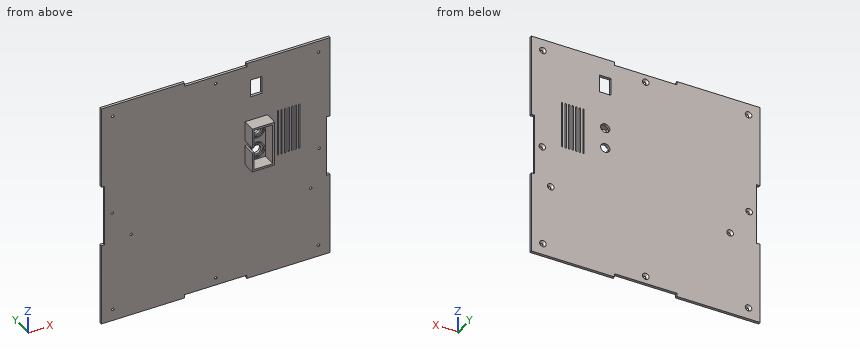
```python
from build123d import *

# Parameters (mm, degrees)
BOSS_EXTRUDE1_DEPTH = 2
SKETCH2_R           = 1
CUT_EXTRUDE1_DEPTH  = 123.699327627
CHAMFER1_SIZE       = 1.5
CUT_EXTRUDE3_DEPTH  = 123.699327627
SKETCH3_W           = 9
SKETCH3_H           = 13.5
CUT_EXTRUDE2_DEPTH  = 123.699327627
SKETCH5_W           = 17
SKETCH5_H           = 34.5
SKETCH5_W_2         = 14
SKETCH5_H_2         = 31.5
BOSS_EXTRUDE2_DEPTH = 10
SKETCH7_R           = 3.5
CUT_EXTRUDE5_DEPTH  = 124.089906166
SKETCH6_W           = 1.5
SKETCH6_H           = 4
CUT_EXTRUDE4_DEPTH  = 10
SKETCH8_R           = 6
SKETCH8_R_2         = 5
BOSS_EXTRUDE3_DEPTH = 1


with BuildPart() as part:
    # Sketch1 → Boss-Extrude1 (new body)
    with BuildSketch(Plane(origin=(0, 0, 0), x_dir=(1, 0, 0), z_dir=(0, 1, 0))):
        Polygon((23.65, -86.75), (86.75, -86.75), (86.75, -23.65), (84.15, -23.65), (84.15, 23.65), (86.75, 23.65), (86.75, 86.75), (23.65, 86.75), (23.65, 84.15), (-23.65, 84.15), (-23.65, 86.75), (-86.75, 86.75), (-86.75, 23.65), (-84.15, 23.65), (-84.15, -23.65), (-86.75, -23.65), (-86.75, -86.75), (-23.65, -86.75), (-23.65, -84.15), (23.65, -84.15), align=None)
    extrude(amount=BOSS_EXTRUDE1_DEPTH)

    # Sketch2 → Cut-Extrude1 (cut, through all)
    with BuildSketch(Plane.XZ):
        with Locations(Location((-77.928932188, 77.928932188, 0), (0, 0, 270))):
            Circle(SKETCH2_R)
        with Locations(Location((0, 78.4, 0), (0, 0, 270))):
            Circle(SKETCH2_R)
        with Locations(Location((77.928932188, 77.928932188, 0), (0, 0, 270))):
            Circle(SKETCH2_R)
        with Locations(Location((-78.4, 0, 0), (0, 0, 270))):
            Circle(SKETCH2_R)
        with Locations(Location((78.4, 0, 0), (0, 0, 270))):
            Circle(SKETCH2_R)
        with Locations(Location((72, -30, 0), (0, 0, 270))):
            Circle(SKETCH2_R)
        with Locations(Location((-64, -22, 0), (0, 0, 270))):
            Circle(SKETCH2_R)
        with Locations(Location((-77.928932188, -77.928932188, 0), (0, 0, 270))):
            Circle(SKETCH2_R)
        with Locations(Location((0, -78.4, 0), (0, 0, 270))):
            Circle(SKETCH2_R)
        with Locations(Location((77.928932188, -77.928932188, 0), (0, 0, 270))):
            Circle(SKETCH2_R)
    extrude(amount=-CUT_EXTRUDE1_DEPTH, mode=Mode.SUBTRACT)

    # Chamfer1
    chamfer1_edges = [part.edges().sort_by_distance(p)[0] for p in [
        (-77.928932188, 2, 78.928932188),
        (0, 2, 79.4),
        (77.928932188, 2, 78.928932188),
        (-78.4, 2, 1),
        (78.4, 2, 1),
        (72, 2, -29),
        (-64, 2, -21),
        (-77.928932188, 2, -76.928932188),
        (0, 2, -77.4),
        (77.928932188, 2, -76.928932188),
    ]]
    chamfer(chamfer1_edges, length=CHAMFER1_SIZE)

    # Sketch4 → Cut-Extrude3 (cut, through all)
    with BuildSketch(Plane.XZ):
        with BuildLine():
            Line((47.7, 40.5), (47.7, 5.5))
            ThreePointArc((47.7, 5.5), (47.2, 5), (46.7, 5.5))
            Line((46.7, 5.5), (46.7, 40.5))
            ThreePointArc((46.7, 40.5), (47.2, 41), (47.7, 40.5))
        make_face()
        with BuildLine():
            Line((50.4, 40.5), (50.4, 5.5))
            ThreePointArc((50.4, 5.5), (49.9, 5), (49.4, 5.5))
            Line((49.4, 5.5), (49.4, 40.5))
            ThreePointArc((49.4, 40.5), (49.9, 41), (50.4, 40.5))
        make_face()
        with BuildLine():
            Line((53.1, 40.5), (53.1, 5.5))
            ThreePointArc((53.1, 5.5), (52.6, 5), (52.1, 5.5))
            Line((52.1, 5.5), (52.1, 40.5))
            ThreePointArc((52.1, 40.5), (52.6, 41), (53.1, 40.5))
        make_face()
        with BuildLine():
            Line((55.8, 40.5), (55.8, 5.5))
            ThreePointArc((55.8, 5.5), (55.3, 5), (54.8, 5.5))
            Line((54.8, 5.5), (54.8, 40.5))
            ThreePointArc((54.8, 40.5), (55.3, 41), (55.8, 40.5))
        make_face()
        with BuildLine():
            Line((58.5, 40.5), (58.5, 5.5))
            ThreePointArc((58.5, 5.5), (58, 5), (57.5, 5.5))
            Line((57.5, 5.5), (57.5, 40.5))
            ThreePointArc((57.5, 40.5), (58, 41), (58.5, 40.5))
        make_face()
        with BuildLine():
            Line((61.2, 40.5), (61.2, 5.5))
            ThreePointArc((61.2, 5.5), (60.7, 5), (60.2, 5.5))
            Line((60.2, 5.5), (60.2, 40.5))
            ThreePointArc((60.2, 40.5), (60.7, 41), (61.2, 40.5))
        make_face()
        with BuildLine():
            Line((63.9, 40.5), (63.9, 5.5))
            ThreePointArc((63.9, 5.5), (63.4, 5), (62.9, 5.5))
            Line((62.9, 5.5), (62.9, 40.5))
            ThreePointArc((62.9, 40.5), (63.4, 41), (63.9, 40.5))
        make_face()
    extrude(amount=-CUT_EXTRUDE3_DEPTH, mode=Mode.SUBTRACT)

    # Sketch3 → Cut-Extrude2 (cut, through all)
    with BuildSketch(Plane.XZ):
        with Locations((30.7, 65.75)):
            Rectangle(SKETCH3_W, SKETCH3_H)
    extrude(amount=-CUT_EXTRUDE2_DEPTH, mode=Mode.SUBTRACT)

    # Sketch5 → Boss-Extrude2 (add)
    with BuildSketch(Plane.XZ):
        with Locations((30.7, 23)):
            Rectangle(SKETCH5_W, SKETCH5_H)
        with Locations((30.7, 23)):
            Rectangle(SKETCH5_W_2, SKETCH5_H_2, mode=Mode.SUBTRACT)
    extrude(amount=BOSS_EXTRUDE2_DEPTH)

    # Sketch7 → Cut-Extrude5 (cut, through all)
    with BuildSketch(Plane.XZ):
        with Locations(Location((30.7, 15, 0), (0, 0, 270))):
            Circle(SKETCH7_R)
        with Locations(Location((30.7, 31, 0), (0, 0, 270))):
            Circle(SKETCH7_R)
    extrude(amount=-CUT_EXTRUDE5_DEPTH, mode=Mode.SUBTRACT)

    # Sketch6 → Cut-Extrude4 (cut)
    with BuildSketch(Plane.XZ.offset(10)):
        with Locations((22.95, 23)):
            Rectangle(SKETCH6_W, SKETCH6_H)
    extrude(amount=-CUT_EXTRUDE4_DEPTH, mode=Mode.SUBTRACT)

    # Sketch8 → Boss-Extrude3 (add)
    # profile 1 of 2: a face of its own
    with BuildSketch(Plane.XZ):
        with Locations(Location((30.7, 31, 0), (0, 0, 90))):
            Circle(SKETCH8_R)
        with Locations(Location((30.7, 31, 0), (0, 0, 270))):
            Circle(SKETCH8_R_2, mode=Mode.SUBTRACT)
    # profile 2 of 2: a face of its own
    with BuildSketch(Plane.XZ):
        with Locations(Location((30.7, 15, 0), (0, 0, 90))):
            Circle(SKETCH8_R)
        with Locations(Location((30.7, 15, 0), (0, 0, 270))):
            Circle(SKETCH8_R_2, mode=Mode.SUBTRACT)
    extrude(amount=BOSS_EXTRUDE3_DEPTH)


solid = part.part
```
Geometry check sheet. Reference: the model listing, model coordinates, mm. Coordinates: 2 decimals unless noted, no trailing zeros. Order: outer loops, then holes, each group sorted by start corner. A loop starts at its lowest first (then second) coordinate and runs counter-clockwise, first axis right, second up. Notation, with made-up numbers: (82, 39) - (107, 39) arc R12 cw to (107, 43) - close; hole circle Ø10 at (-28, 23). An arc over 180 degrees is marked (long way). Answer as a JSON object with one key per item and string values. Group by question number.
Item 1: Sectioned sample at A-A, the plane z = 63. Record the cut outline in (x, y), and give its area (3 significant figures).
Item 2: Scan lines: probe 1 along Z at (x, y) = (22.5, -8); probe 2 along X at (y, z) = (0.2, -30); probe 3 along Z at (x, y) = (78.4, 0.4). Record each from-to range of solid material in increasing order.
Item 3: Sectioned sample at D-D, the plane x = -9. Record the cut outline in (y, z), and give its area (3 significant figures).
Item 4: Sectioned sample at B-B, the plane y = -4.75. Record the cut outline in (x, z), and give its area (4 significant figures).
Item 5: Sectioned sample at C-C, the plane z = 31. Give the number of separate pieces and of enclosed holes in the cut face, and give its area (3 significant figures).
Item 6: Depth check by flat-ended pin: pin 1 Ø0.6 at (x, y) = (-10, 0.5) entering from -Z; pin 2 Ø1.6 at (y, z) = (1, 18.5) entering from +X; pin 3 Ø1.2 at (x, z) = (-78.4, 0) entering from -Y; pin 4 Ø3 at (x, y) = (33.5, -4.5) entering from -Z. Enter the tip coordinate at first touch or a pass-through.
Resolved:
{
 "1": {"outline": "(-86.75, 0) - (26.2, 0) - (26.2, 2) - (-86.75, 2) - close; (35.2, 0) - (86.75, 0) - (86.75, 2) - (35.2, 2) - close", "area": "329 mm^2"},
 "2": {"probe 1": "5.75 to 21, 25 to 40.25", "probe 2": "-86.75 to 71, 73 to 86.75", "probe 3": "-86.75 to -78.81, -77.05 to -1, 1 to 77.05, 78.81 to 86.75"},
 "3": {"outline": "(0, -84.15) - (2, -84.15) - (2, 84.15) - (0, 84.15) - close", "area": "337 mm^2"},
 "4": {"outline": "(22.2, 5.75) - (39.2, 5.75) - (39.2, 40.25) - (22.2, 40.25) - (22.2, 25) - (23.7, 25) - (23.7, 38.75) - (37.7, 38.75) - (37.7, 7.25) - (23.7, 7.25) - (23.7, 21) - (22.2, 21) - close", "area": "139.5 mm^2"},
 "5": {"separate pieces": "9", "enclosed holes": "0", "area": "351 mm^2"},
 "6": {"pin 1": "z = -84.15", "pin 2": "x = 84.15", "pin 3": "through", "pin 4": "z = 5.75"}
}
